Verification items for the finished model (mm, model axes). Give positions to 0.01 mm unless a question says otherwise; leave off trailing zeros. Write each loop counter-clockwise with the first axis right and the second up, starting at its lowest first coordinate (ties: lowest second). Pieces come first, ordered by that corner, then holes. Notation, with made-up numbers: (82, 42) -> (116, 42) arc R23 cw to (116, 78) -> close; hole circle Ø7 at (-35, 44). An arc over 180 degrees is marked (long way). Write item = value, one per line.
from build123d import *

# Parameters (mm, degrees)
TABAN_FLAN_1_DEPTH = 10


# Sheet-metal steps are written as plain solids
with BuildPart() as part:
    # Çizim1 → Taban-Flanş1 (new body)
    with BuildSketch(Plane.XY):
        with BuildLine():
            Line((0, 0), (0, 370))
            ThreePointArc((0, 370), (241.280287234, 425.036333585), (485, 468))
            Line((485, 468), (485, -54))
            Line((485, -54), (454, -54))
            Line((454, -54), (454, 0))
            Line((454, 0), (0, 0))
        make_face()
    extrude(amount=-TABAN_FLAN_1_DEPTH)


solid = part.part
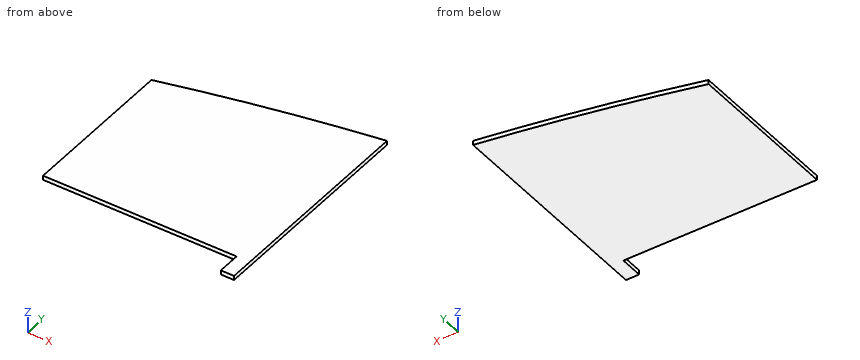
Item 1: Sectioned sample at C-C on x = 283.5. Record the cut outline in (y, z), then the cut area to 3 significant figures.
Response values:
outline = (0, -10) -> (433.38, -10) -> (433.38, 0) -> (0, 0) -> close
area = 4,330 mm^2
Item 2: Sectioned sample at A-A on z = -1.5. Record the cut outline in (x, y), then the cut area to 3 significant figures.
Response values:
outline = (0, 0) -> (454, 0) -> (454, -54) -> (485, -54) -> (485, 468) arc R4972.55 ccw to (0, 370) -> close
area = 207,000 mm^2
Item 3: Go/stop test with flat-tipped pins: P1, Ø3, axis at x = 194.5, z = -4.5, coming from the -Y side; P2, Ø1, axis at x = 185, z = -3, coming from the +Y side; P3, Ø3, axis at y = -26.5, z = -6, coming from the -X side. Record where each tip stops, or that it passes through.
Response values:
P1 = 0
P2 = 413.43
P3 = 454
Item 4: Material ranges on line 1 (X direction, y = -32, z = -9); line 2 (Y direction, x = 242, z = -2); line 3 (Y direction, x = 448.5, z = -2.5), recorded low to high.
Response values:
line_1 = 454 to 485
line_2 = 0 to 425.18
line_3 = 0 to 462.36
